Source: CAD feature listing. Evaluate the final solid. Frame: model axes, mm. A direction names the side the tool comes from. Round coordinates to 2 decimals unless told otherwise and drop trailing zeros. Order: outer loops, then holes, each group sorted by start corner. A loop starts at its lowest first (then second) coordinate and runs counter-clockwise, first axis right, second up. Notation, with made-up numbers: M 81.25,-10 L 95.25,-10 A19 ccw 95.25,16 Z; hole C 82.25,15.25 d1. An arc over 180 degrees is marked long. Answer in a Markdown table with one row per item. Add a question column.
```python
from build123d import *

# Parameters (mm, degrees)
NAME_PLATE_BEZEL_DEPTH     = 3
NAME_PLATE_BACKPLATE_DEPTH = 1
HOLE_BEZEL_DEPTH           = 2.25
HOLE_BEZEL_DEPTH_BACK      = 0.75
HOLE_SKETCH_R              = 4
HOLE_SKETCH_R_2            = 2.5
HOLE_CUTOUT_DEPTH          = 57.740637994
HOLE_CUTOUT_DEPTH_BACK     = 57.740637994
HOLE_SKETCH_6_R            = 2.5


with BuildPart() as part:
    # Base Plate Sketch → Name Plate Bezel (new body)
    with BuildSketch(Plane.XY):
        with BuildLine():
            Line((-42.549751124, 15.5), (42.549751124, 15.5))
            ThreePointArc((42.549751124, 15.5), (44.689893576, 14.829332766), (46.064530205, 13.057221485))
            ThreePointArc((46.064530205, 13.057221485), (48.321727581, 9.650169967), (51.852941176, 7.592630032))
            ThreePointArc((51.852941176, 7.592630032), (53.76649875, 6.236327413), (54.5, 4.008495442))
            Line((54.5, 4.008495442), (54.5, -4.008495442))
            ThreePointArc((54.5, -4.008495442), (53.76649875, -6.236327413), (51.852941176, -7.592630032))
            ThreePointArc((51.852941176, -7.592630032), (48.321727581, -9.650169967), (46.064530205, -13.057221485))
            ThreePointArc((46.064530205, -13.057221485), (44.689893576, -14.829332766), (42.549751124, -15.5))
            Line((42.549751124, -15.5), (-42.549751124, -15.5))
            ThreePointArc((-42.549751124, -15.5), (-44.689893576, -14.829332766), (-46.064530205, -13.057221485))
            ThreePointArc((-46.064530205, -13.057221485), (-48.321727581, -9.650169967), (-51.852941176, -7.592630032))
            ThreePointArc((-51.852941176, -7.592630032), (-53.76649875, -6.236327413), (-54.5, -4.008495442))
            Line((-54.5, -4.008495442), (-54.5, 4.008495442))
            ThreePointArc((-54.5, 4.008495442), (-53.76649875, 6.236327413), (-51.852941176, 7.592630032))
            ThreePointArc((-51.852941176, 7.592630032), (-48.321727581, 9.650169967), (-46.064530205, 13.057221485))
            ThreePointArc((-46.064530205, 13.057221485), (-44.689893576, 14.829332766), (-42.549751124, 15.5))
        make_face()
        with BuildLine():
            Line((-42.549751124, 14), (42.549751124, 14))
            ThreePointArc((42.549751124, 14), (43.833836595, 13.59759966), (44.658618573, 12.534332891))
            ThreePointArc((44.658618573, 12.534332891), (47.292015511, 8.559439453), (51.411764706, 6.158976196))
            ThreePointArc((51.411764706, 6.158976196), (52.55989925, 5.345194625), (53, 4.008495442))
            Line((53, 4.008495442), (53, -4.008495442))
            ThreePointArc((53, -4.008495442), (52.55989925, -5.345194625), (51.411764706, -6.158976196))
            ThreePointArc((51.411764706, -6.158976196), (47.292015511, -8.559439453), (44.658618573, -12.534332891))
            ThreePointArc((44.658618573, -12.534332891), (43.833836595, -13.59759966), (42.549751124, -14))
            Line((42.549751124, -14), (-42.549751124, -14))
            ThreePointArc((-42.549751124, -14), (-43.833836595, -13.59759966), (-44.658618573, -12.534332891))
            ThreePointArc((-44.658618573, -12.534332891), (-47.292015511, -8.559439453), (-51.411764706, -6.158976196))
            ThreePointArc((-51.411764706, -6.158976196), (-52.55989925, -5.345194625), (-53, -4.008495442))
            Line((-53, -4.008495442), (-53, 4.008495442))
            ThreePointArc((-53, 4.008495442), (-52.55989925, 5.345194625), (-51.411764706, 6.158976196))
            ThreePointArc((-51.411764706, 6.158976196), (-47.292015511, 8.559439453), (-44.658618573, 12.534332891))
            ThreePointArc((-44.658618573, 12.534332891), (-43.833836595, 13.59759966), (-42.549751124, 14))
        make_face(mode=Mode.SUBTRACT)
    extrude(amount=NAME_PLATE_BEZEL_DEPTH)

    # Sketch1<6> → Name Plate Backplate (add)
    with BuildSketch(Plane.XY):
        with BuildLine():
            Line((-42.549751124, 15.5), (42.549751124, 15.5))
            ThreePointArc((42.549751124, 15.5), (44.689893576, 14.829332766), (46.064530205, 13.057221485))
            ThreePointArc((46.064530205, 13.057221485), (48.321727581, 9.650169967), (51.852941176, 7.592630032))
            ThreePointArc((51.852941176, 7.592630032), (53.76649875, 6.236327413), (54.5, 4.008495442))
            Line((54.5, 4.008495442), (54.5, -4.008495442))
            ThreePointArc((54.5, -4.008495442), (53.76649875, -6.236327413), (51.852941176, -7.592630032))
            ThreePointArc((51.852941176, -7.592630032), (48.321727581, -9.650169967), (46.064530205, -13.057221485))
            ThreePointArc((46.064530205, -13.057221485), (44.689893576, -14.829332766), (42.549751124, -15.5))
            Line((42.549751124, -15.5), (-42.549751124, -15.5))
            ThreePointArc((-42.549751124, -15.5), (-44.689893576, -14.829332766), (-46.064530205, -13.057221485))
            ThreePointArc((-46.064530205, -13.057221485), (-48.321727581, -9.650169967), (-51.852941176, -7.592630032))
            ThreePointArc((-51.852941176, -7.592630032), (-53.76649875, -6.236327413), (-54.5, -4.008495442))
            Line((-54.5, -4.008495442), (-54.5, 4.008495442))
            ThreePointArc((-54.5, 4.008495442), (-53.76649875, 6.236327413), (-51.852941176, 7.592630032))
            ThreePointArc((-51.852941176, 7.592630032), (-48.321727581, 9.650169967), (-46.064530205, 13.057221485))
            ThreePointArc((-46.064530205, 13.057221485), (-44.689893576, 14.829332766), (-42.549751124, 15.5))
        make_face()
    extrude(amount=NAME_PLATE_BACKPLATE_DEPTH)

    # Hole Sketch → Hole Bezel (add, two sides: drawn at the far end of the back side and taken through both)
    # profile 1 of 2: a face of its own
    with BuildSketch(Plane.XY.offset(-HOLE_BEZEL_DEPTH_BACK)):
        with Locations((45.5, 0)):
            Circle(HOLE_SKETCH_R)
        with Locations((45.5, 0)):
            Circle(HOLE_SKETCH_R_2, mode=Mode.SUBTRACT)
    # profile 2 of 2: a face of its own
    with BuildSketch(Plane.XY.offset(-HOLE_BEZEL_DEPTH_BACK)):
        with Locations((-45.5, 0)):
            Circle(HOLE_SKETCH_R)
        with Locations((-45.5, 0)):
            Circle(HOLE_SKETCH_R_2, mode=Mode.SUBTRACT)
    extrude(amount=HOLE_BEZEL_DEPTH + HOLE_BEZEL_DEPTH_BACK)

    # Hole Sketch<6> → Hole Cutout (cut, two sides: drawn at the far end of the back side and taken through both)
    with BuildSketch(Plane.XY.offset(-HOLE_CUTOUT_DEPTH_BACK)):
        with Locations((-45.5, 0)):
            Circle(HOLE_SKETCH_6_R)
        with Locations((45.5, 0)):
            Circle(HOLE_SKETCH_6_R)
    extrude(amount=HOLE_CUTOUT_DEPTH + HOLE_CUTOUT_DEPTH_BACK, mode=Mode.SUBTRACT)


solid = part.part
```
(1) Draft query along X for faces 4 (the face through (-46, -3, 2.25)), 5 (the face through (0, 15, 3)), 6 (the face through (-53.786, 6.209, 1.479)). Return one class per face: +X half, -X half, draft (parallel to the pull), parting line (faces both ways), or undercut.
(2) Cut plane A-A (y = 0). Count the separate pieces of the cut face and the enclosed holes in it, and give its area (3 significant figures).
(3) Pin query (flat end, axial travel): pin 1 (9.5 mm diameter, centred on x = -19, y = 7.5, fed in from -Z); pin 2 (9 mm diameter, centred on x = 45, y = -1, fed in from +Z); pin 3 (2 mm diameter, centred on y = -9.5, z = 2.5, fed in from +X); pin 4 (4.5 mm diameter, centred on x = -45.5, y = 0, fed in from -Z). Return the tip coordinate at first contact, or that it passes through.
(4) Line query: line 1 (Y direction, x = -45.5, z = -0.05); line 2 (Y direction, x = -42, z = 1.3); line 3 (Y direction, x = 30, z = 2.75). Output: solid intervals per line, ascending. Write a range as from..to.
(5) Cut plane B-B (x = -15.5). Return loops of the section in (y, z).
(6) Access query for faces 1 (the face through (-46, -3, -0.75)), 2 (the face through (42.3, -2.4, -0.4)), 3 (the face through (42.3, -2.4, 1.6)). Directions: +Z, -Z, +X, -X, +Y, -Y. A direction counts if a zero-diameter tool reaches every point of the face in a straight line with its end or side. Return the directions, or none.
Answer list:
| question | item | result |
|---|---|---|
| 1 | face 4 | undercut |
| 1 | face 5 | draft |
| 1 | face 6 | -X half |
| 2 | separate pieces | 3 |
| 2 | enclosed holes | 0 |
| 2 | area | 117 mm² |
| 3 | pin 1 | z = 0 |
| 3 | pin 2 | z = 2.25 |
| 3 | pin 3 | x = 49.83 |
| 3 | pin 4 | through |
| 4 | line 1 | -4..-2.5, 2.5..4 |
| 4 | line 2 | -15.5..-14, -1.94..1.94, 14..15.5 |
| 4 | line 3 | -15.5..-14, 14..15.5 |
| 5 | outline | M -15.5,0 L 15.5,0 L 15.5,3 L 14,3 L 14,1 L -14,1 L -14,3 L -15.5,3 Z |
| 6 | face 1 | -Z, +X, -X, +Y, -Y |
| 6 | face 2 | -Z |
| 6 | face 3 | +Z |
